Geometry: final body of the model. Coordinates: model frame, mm. A direction names the side the tool comes from. Coordinates: 2 decimals unless noted, no trailing zeros. Use one line per item in the form item = value.
```python
from build123d import *

# Parameters (mm, degrees)
SKETCH4_W                                     = 200
SKETCH4_H                                     = 100
BOSS_EXTRUDE1_DEPTH                           = 10
CBORE_FOR_M6_HEX_HEAD_CAP_SCREW7_D            = 6
CBORE_FOR_M6_HEX_HEAD_CAP_SCREW7_DEPTH        = 8
CBORE_FOR_M6_HEX_HEAD_CAP_SCREW7_CBORE_D      = 8
CBORE_FOR_M6_HEX_HEAD_CAP_SCREW7_CBORE_DEPTH  = 2
CBORE_FOR_M6_HEX_HEAD_CAP_SCREW7_TIP          = 1.802581857
CBORE_FOR_M6_HEX_HEAD_CAP_SCREW8_D            = 6
CBORE_FOR_M6_HEX_HEAD_CAP_SCREW8_DEPTH        = 8
CBORE_FOR_M6_HEX_HEAD_CAP_SCREW8_CBORE_D      = 8
CBORE_FOR_M6_HEX_HEAD_CAP_SCREW8_CBORE_DEPTH  = 2
CBORE_FOR_M6_HEX_HEAD_CAP_SCREW8_TIP          = 1.802581857
CBORE_FOR_M6_HEX_HEAD_CAP_SCREW9_D            = 6
CBORE_FOR_M6_HEX_HEAD_CAP_SCREW9_DEPTH        = 8
CBORE_FOR_M6_HEX_HEAD_CAP_SCREW9_CBORE_D      = 8
CBORE_FOR_M6_HEX_HEAD_CAP_SCREW9_CBORE_DEPTH  = 2
CBORE_FOR_M6_HEX_HEAD_CAP_SCREW9_TIP          = 1.802581857
CBORE_FOR_M6_HEX_HEAD_CAP_SCREW10_D           = 6
CBORE_FOR_M6_HEX_HEAD_CAP_SCREW10_DEPTH       = 8
CBORE_FOR_M6_HEX_HEAD_CAP_SCREW10_CBORE_D     = 8
CBORE_FOR_M6_HEX_HEAD_CAP_SCREW10_CBORE_DEPTH = 2
CBORE_FOR_M6_HEX_HEAD_CAP_SCREW10_TIP         = 1.802581857
F_1_0_1_DIAMETER_HOLE7_D                      = 5
F_1_0_1_DIAMETER_HOLE7_DEPTH                  = 8
F_1_0_1_DIAMETER_HOLE7_TIP                    = 1.502151548
F_1_0_1_DIAMETER_HOLE8_D                      = 5
F_1_0_1_DIAMETER_HOLE8_DEPTH                  = 8
F_1_0_1_DIAMETER_HOLE8_TIP                    = 1.502151548
F_1_0_1_DIAMETER_HOLE9_D                      = 5
F_1_0_1_DIAMETER_HOLE9_DEPTH                  = 8
F_1_0_1_DIAMETER_HOLE9_TIP                    = 1.502151548
F_1_0_1_DIAMETER_HOLE10_D                     = 5
F_1_0_1_DIAMETER_HOLE10_DEPTH                 = 8
F_1_0_1_DIAMETER_HOLE10_TIP                   = 1.502151548
F_5_0_5_DIAMETER_HOLE1_D                      = 5
F_5_0_5_DIAMETER_HOLE1_DEPTH                  = 8
F_5_0_5_DIAMETER_HOLE1_TIP                    = 1.502151548
F_5_0_5_DIAMETER_HOLE2_D                      = 5
F_5_0_5_DIAMETER_HOLE2_DEPTH                  = 8
F_5_0_5_DIAMETER_HOLE2_TIP                    = 1.502151548
F_5_0_5_DIAMETER_HOLE3_D                      = 5
F_5_0_5_DIAMETER_HOLE3_DEPTH                  = 8
F_5_0_5_DIAMETER_HOLE3_TIP                    = 1.502151548
F_5_0_5_DIAMETER_HOLE5_D                      = 5
F_5_0_5_DIAMETER_HOLE5_DEPTH                  = 8
F_5_0_5_DIAMETER_HOLE5_TIP                    = 1.502151548
FILLET1_R                                     = 10
FILLET2_R                                     = 10
FILLET3_R                                     = 10
FILLET4_R                                     = 10
SCALE2_SCALE                                  = 1.5
SCALE6_SCALE                                  = 0.935
SCALE7_SCALE                                  = 0.9


with BuildPart() as part:
    # Sketch4 → Boss-Extrude1 (new body)
    with BuildSketch(Plane.XY):
        with Locations((100, 50)):
            Rectangle(SKETCH4_W, SKETCH4_H)
    extrude(amount=BOSS_EXTRUDE1_DEPTH)

    # CBORE for M6 Hex Head Cap Screw7
    with Locations(Plane(origin=(0, 0, 0), x_dir=(-1, 0, 0), z_dir=(0, 0, -1))):
        with Locations((-80, 83.464013217)):
            CounterBoreHole(CBORE_FOR_M6_HEX_HEAD_CAP_SCREW7_D / 2, CBORE_FOR_M6_HEX_HEAD_CAP_SCREW7_CBORE_D / 2, CBORE_FOR_M6_HEX_HEAD_CAP_SCREW7_CBORE_DEPTH, depth=CBORE_FOR_M6_HEX_HEAD_CAP_SCREW7_DEPTH)
            with Locations((0, 0, -(CBORE_FOR_M6_HEX_HEAD_CAP_SCREW7_DEPTH + CBORE_FOR_M6_HEX_HEAD_CAP_SCREW7_TIP / 2))):  # 118° drill point
                Cone(0, CBORE_FOR_M6_HEX_HEAD_CAP_SCREW7_D / 2, CBORE_FOR_M6_HEX_HEAD_CAP_SCREW7_TIP, mode=Mode.SUBTRACT)

    # CBORE for M6 Hex Head Cap Screw8
    with Locations(Plane(origin=(0, 0, 0), x_dir=(-1, 0, 0), z_dir=(0, 0, -1))):
        with Locations((-20, 83.464013217)):
            CounterBoreHole(CBORE_FOR_M6_HEX_HEAD_CAP_SCREW8_D / 2, CBORE_FOR_M6_HEX_HEAD_CAP_SCREW8_CBORE_D / 2, CBORE_FOR_M6_HEX_HEAD_CAP_SCREW8_CBORE_DEPTH, depth=CBORE_FOR_M6_HEX_HEAD_CAP_SCREW8_DEPTH)
            with Locations((0, 0, -(CBORE_FOR_M6_HEX_HEAD_CAP_SCREW8_DEPTH + CBORE_FOR_M6_HEX_HEAD_CAP_SCREW8_TIP / 2))):  # 118° drill point
                Cone(0, CBORE_FOR_M6_HEX_HEAD_CAP_SCREW8_D / 2, CBORE_FOR_M6_HEX_HEAD_CAP_SCREW8_TIP, mode=Mode.SUBTRACT)

    # CBORE for M6 Hex Head Cap Screw9
    with Locations(Plane(origin=(0, 0, 0), x_dir=(-1, 0, 0), z_dir=(0, 0, -1))):
        with Locations((-20, 16.814013217)):
            CounterBoreHole(CBORE_FOR_M6_HEX_HEAD_CAP_SCREW9_D / 2, CBORE_FOR_M6_HEX_HEAD_CAP_SCREW9_CBORE_D / 2, CBORE_FOR_M6_HEX_HEAD_CAP_SCREW9_CBORE_DEPTH, depth=CBORE_FOR_M6_HEX_HEAD_CAP_SCREW9_DEPTH)
            with Locations((0, 0, -(CBORE_FOR_M6_HEX_HEAD_CAP_SCREW9_DEPTH + CBORE_FOR_M6_HEX_HEAD_CAP_SCREW9_TIP / 2))):  # 118° drill point
                Cone(0, CBORE_FOR_M6_HEX_HEAD_CAP_SCREW9_D / 2, CBORE_FOR_M6_HEX_HEAD_CAP_SCREW9_TIP, mode=Mode.SUBTRACT)

    # CBORE for M6 Hex Head Cap Screw10
    with Locations(Plane(origin=(0, 0, 0), x_dir=(-1, 0, 0), z_dir=(0, 0, -1))):
        with Locations((-80, 16.814013217)):
            CounterBoreHole(CBORE_FOR_M6_HEX_HEAD_CAP_SCREW10_D / 2, CBORE_FOR_M6_HEX_HEAD_CAP_SCREW10_CBORE_D / 2, CBORE_FOR_M6_HEX_HEAD_CAP_SCREW10_CBORE_DEPTH, depth=CBORE_FOR_M6_HEX_HEAD_CAP_SCREW10_DEPTH)
            with Locations((0, 0, -(CBORE_FOR_M6_HEX_HEAD_CAP_SCREW10_DEPTH + CBORE_FOR_M6_HEX_HEAD_CAP_SCREW10_TIP / 2))):  # 118° drill point
                Cone(0, CBORE_FOR_M6_HEX_HEAD_CAP_SCREW10_D / 2, CBORE_FOR_M6_HEX_HEAD_CAP_SCREW10_TIP, mode=Mode.SUBTRACT)

    # Ø1.0 (1) Diameter Hole7
    with Locations(Plane.XY.offset(10)):
        with Locations((20, 75.196019825)):
            Hole(F_1_0_1_DIAMETER_HOLE7_D / 2, depth=F_1_0_1_DIAMETER_HOLE7_DEPTH)
            with Locations((0, 0, -(F_1_0_1_DIAMETER_HOLE7_DEPTH + F_1_0_1_DIAMETER_HOLE7_TIP / 2))):  # 118° drill point
                Cone(0, F_1_0_1_DIAMETER_HOLE7_D / 2, F_1_0_1_DIAMETER_HOLE7_TIP, mode=Mode.SUBTRACT)

    # Ø1.0 (1) Diameter Hole8
    with Locations(Plane.XY.offset(10)):
        with Locations((80, 75.196019825)):
            Hole(F_1_0_1_DIAMETER_HOLE8_D / 2, depth=F_1_0_1_DIAMETER_HOLE8_DEPTH)
            with Locations((0, 0, -(F_1_0_1_DIAMETER_HOLE8_DEPTH + F_1_0_1_DIAMETER_HOLE8_TIP / 2))):  # 118° drill point
                Cone(0, F_1_0_1_DIAMETER_HOLE8_D / 2, F_1_0_1_DIAMETER_HOLE8_TIP, mode=Mode.SUBTRACT)

    # Ø1.0 (1) Diameter Hole9
    with Locations(Plane.XY.offset(10)):
        with Locations((20, 25.221019825)):
            Hole(F_1_0_1_DIAMETER_HOLE9_D / 2, depth=F_1_0_1_DIAMETER_HOLE9_DEPTH)
            with Locations((0, 0, -(F_1_0_1_DIAMETER_HOLE9_DEPTH + F_1_0_1_DIAMETER_HOLE9_TIP / 2))):  # 118° drill point
                Cone(0, F_1_0_1_DIAMETER_HOLE9_D / 2, F_1_0_1_DIAMETER_HOLE9_TIP, mode=Mode.SUBTRACT)

    # Ø1.0 (1) Diameter Hole10
    with Locations(Plane.XY.offset(10)):
        with Locations((80, 25.221019825)):
            Hole(F_1_0_1_DIAMETER_HOLE10_D / 2, depth=F_1_0_1_DIAMETER_HOLE10_DEPTH)
            with Locations((0, 0, -(F_1_0_1_DIAMETER_HOLE10_DEPTH + F_1_0_1_DIAMETER_HOLE10_TIP / 2))):  # 118° drill point
                Cone(0, F_1_0_1_DIAMETER_HOLE10_D / 2, F_1_0_1_DIAMETER_HOLE10_TIP, mode=Mode.SUBTRACT)

    # Ø5.0 (5) Diameter Hole1
    with Locations(Plane.XY.offset(10)):
        with Locations((120, 90)):
            Hole(F_5_0_5_DIAMETER_HOLE1_D / 2, depth=F_5_0_5_DIAMETER_HOLE1_DEPTH)
            with Locations((0, 0, -(F_5_0_5_DIAMETER_HOLE1_DEPTH + F_5_0_5_DIAMETER_HOLE1_TIP / 2))):  # 118° drill point
                Cone(0, F_5_0_5_DIAMETER_HOLE1_D / 2, F_5_0_5_DIAMETER_HOLE1_TIP, mode=Mode.SUBTRACT)

    # Ø5.0 (5) Diameter Hole2
    with Locations(Plane.XY.offset(10)):
        with Locations((180, 90)):
            Hole(F_5_0_5_DIAMETER_HOLE2_D / 2, depth=F_5_0_5_DIAMETER_HOLE2_DEPTH)
            with Locations((0, 0, -(F_5_0_5_DIAMETER_HOLE2_DEPTH + F_5_0_5_DIAMETER_HOLE2_TIP / 2))):  # 118° drill point
                Cone(0, F_5_0_5_DIAMETER_HOLE2_D / 2, F_5_0_5_DIAMETER_HOLE2_TIP, mode=Mode.SUBTRACT)

    # Ø5.0 (5) Diameter Hole3
    with Locations(Plane.XY.offset(10)):
        with Locations((120, 43.628026433)):
            Hole(F_5_0_5_DIAMETER_HOLE3_D / 2, depth=F_5_0_5_DIAMETER_HOLE3_DEPTH)
            with Locations((0, 0, -(F_5_0_5_DIAMETER_HOLE3_DEPTH + F_5_0_5_DIAMETER_HOLE3_TIP / 2))):  # 118° drill point
                Cone(0, F_5_0_5_DIAMETER_HOLE3_D / 2, F_5_0_5_DIAMETER_HOLE3_TIP, mode=Mode.SUBTRACT)

    # Ø5.0 (5) Diameter Hole5
    with Locations(Plane.XY.offset(10)):
        with Locations((180, 43.628026433)):
            Hole(F_5_0_5_DIAMETER_HOLE5_D / 2, depth=F_5_0_5_DIAMETER_HOLE5_DEPTH)
            with Locations((0, 0, -(F_5_0_5_DIAMETER_HOLE5_DEPTH + F_5_0_5_DIAMETER_HOLE5_TIP / 2))):  # 118° drill point
                Cone(0, F_5_0_5_DIAMETER_HOLE5_D / 2, F_5_0_5_DIAMETER_HOLE5_TIP, mode=Mode.SUBTRACT)

    # Fillet1
    fillet1_edges = [part.edges().sort_by_distance(p)[0] for p in [
        (0, 100, 5),
    ]]
    fillet(fillet1_edges, radius=FILLET1_R)

    # Fillet2
    fillet2_edges = [part.edges().sort_by_distance(p)[0] for p in [
        (0, 0, 5),
    ]]
    fillet(fillet2_edges, radius=FILLET2_R)

    # Fillet3
    fillet3_edges = [part.edges().sort_by_distance(p)[0] for p in [
        (200, 0, 5),
    ]]
    fillet(fillet3_edges, radius=FILLET3_R)

    # Fillet4
    fillet4_edges = [part.edges().sort_by_distance(p)[0] for p in [
        (200, 100, 5),
    ]]
    fillet(fillet4_edges, radius=FILLET4_R)


with BuildPart() as part_1:
    # Scale2: scaled about (100.292046526, 49.941397219, 5.001946843)
    add(part.part.scale(SCALE2_SCALE).moved(Location((-50.146023263, -24.97069861, -2.500973421))))


with BuildPart() as part_2:
    # Scale6: scaled about (100.292046526, 49.941397219, 5.001946844)
    add(part_1.part.scale(SCALE6_SCALE).moved(Location((6.518983024, 3.246190819, 0.325126545))))


with BuildPart() as part_3:
    # Scale7: scaled about (100.292046526, 49.941397219, 5.001946844)
    add(part_2.part.scale(SCALE7_SCALE).moved(Location((10.029204653, 4.994139722, 0.500194684))))


solid = part_3.part
```
1) Section A-A, the plane z = 4. Give the number of separate pieces and of enclosed holes in the cut face, and give its area (3 significant figures).
Results found:
separate_pieces = 1
enclosed_holes = 12
area = 31,300 mm2
2) Access query for faces 5 (the cylindrical face through (78.176, 90.805, 5.053)), 6 (the flat face through (226.148, 49, 5)), 7 (the cylindrical face through (123.47, 44.63, 6.19)). Directions: +Z, -Z, +X, -X, +Y, -Y. A direction counts if a zero-diameter tool reaches every point of the face in a straight line with its end or side. Return the directions, or none.
Results found:
face_5 = -Z
face_6 = +Z, -Z, +X, +Y, -Y
face_7 = +Z
3) Material intervals for probe 1 along X at (y, z) = (41.5, 2.5); probe 2 along X at (y, z) = (89, -0.5); probe 3 along X at (y, z) = (-6.5, 2.5), sorted ascending. Write a range as from..to.
Results found:
probe_1 = -26.3..122.05, 128.29..197.78, 204.02..226.15
probe_2 = -26.3..-4.92, 2.8..70.82, 78.54..226.15
probe_3 = -24.77..224.62
4) Contact query for flat-ended pins moving along their axis: P1, Ø16, axis at x = -1.06, y = 8.13, coming from the -Z side; P2, Ø6, axis at x = -1.06, y = 8.13, coming from the -Z side; P3, Ø7, axis at x = 74.68, y = 92.26, coming from the -Z side; P4, Ø5, axis at x = 0, y = 9.5, coming from the -Z side. Output: stop coordinate, or through.
Results found:
P1 = -1.31
P2 = 9.26
P3 = 8.96
P4 = 1.21
5) Pull-direction query (X, two-part tool) for faces 1 (the cylindrical face through (77.183, 16.818, 6.191)), 2 (the flat face through (98, 113.128, 5)), 3 (the cylindrical face through (204.056, 42.111, 6.191)), 4 (the cylindrical face through (-22.702, 109.332, 5.088)); classes: released by +X, released by -X, zero draft, split by the parting line, or undercut.
Results found:
face_1 = undercut
face_2 = zero draft
face_3 = undercut
face_4 = released by -X
